Build history of the part. All positions in model axes, mm. Give positions to 0.01 mm unless a question says otherwise; leave off trailing zeros. Write each loop counter-clockwise with the first axis right and the second up, starting at its lowest first coordinate (ties: lowest second). Pieces come first, ordered by that corner, then holes. Notation, with made-up numbers: M 39,-17 L 98,-17 A16 ccw 98,-13 Z; hole C 33.5,-5 d1. An arc over 180 degrees is marked long. Return JSON: item names as keys, results as strings. Group by question number.
Q1. Flat gauge pin, fed straight in: pin 1 Ø7 at (x, z) = (0, -36.591) entering from +Y. Where does the tip first touch, or does it go through?
Q2. Band-saw the part on B-B, the plane y = 6. Give the cut face in (x, z), then the cut area to 3 significant figures.
Q3. Band-saw the part on C-C, the plane z = 32. Give the cut face in (x, y).
Q4. Band-saw the part on A-A, the plane x = 0. Give the cut face in (y, z), then the cut area to 3 significant figures.
Q5. Wall check: probe 1 along Z at (x, y) = (0, 5.75); probe 2 along X at (y, z) = (3.5, -32); probe 3 along Z at (x, y) = (4.75, 0.75). Give the ranges that are in metal, low to high.
Q6. Pull direction X, two halves, no side cores. Call faces 1 (the flat face through (-9, 4, -1)), 2 (the cylindrical face through (-3.226, 4.437, -41.65)), 3 (the flat face through (0, 0, 1)): +X half, -X half, draft (parallel to the pull), parting line (faces both ways), or undercut.
Autodesk Inventor part; units mm, degrees
ref_plane "YZ Plane" through (0, 0, 0) normal (1, 0, 0) x (0, 1, 0)
ref_plane "XZ Plane" through (0, 0, 0) normal (0, 1, 0) x (-1, 0, 0)
ref_plane "XY Plane" through (0, 0, 0) normal (0, 0, 1) x (1, 0, 0)
sketch "Sketch1" plane through (0, 0, 0) normal (0, 1, 0) x (-1, 0, 0)
  line L0 (3.6, 44.409) -> (-3.6, 44.409)
  line L1 (-9, 39.009) -> (-9, -39.009)
  line L2 (-3.6, -44.409) -> (3.6, -44.409)
  line L3 (9, -39.009) -> (9, 39.009)
  line L4 (9, 44.409) -> (-9, -44.409) construction
  line L5 (-9, 44.409) -> (9, -44.409) construction
  arc A0 (3.6, -44.409) -> (9, -39.009) centre (3.6, -39.009) ccw
  arc A1 (-9, -39.009) -> (-3.6, -44.409) centre (-3.6, -39.009) ccw
  arc A2 (9, 39.009) -> (3.6, 44.409) centre (3.6, 39.009) ccw
  arc A3 (-3.6, 44.409) -> (-9, 39.009) centre (-3.6, 39.009) ccw
  line L6 (0, -44.409) -> (0, -36.591)
  circle A4 centre (0, -36.591) radius 6
  line L7 (0, 0) -> (1.5436, 0)
  circle A5 centre (0, 36.591) radius 6
  dimension "d0" = 18
  dimension "d1" = 88.818
  dimension "d2" = 5.4
  dimension "d3" = 7.818
  dimension "d4" = 12
extrude "Extrusion1" add sketch "Sketch1" along normal blind 9
properties part number "LegLverr"
From the geometry:
{
 "1": {"pin 1": "passes through"},
 "2": {"outline": "M -9,-39.01 A5.4 ccw -3.6,-44.41 L 3.6,-44.41 A5.4 ccw 9,-39.01 L 9,39.01 A5.4 ccw 3.6,44.41 L -3.6,44.41 A5.4 ccw -9,39.01 Z; hole C 0,-36.59 d12; hole C 0,36.59 d12", "area": "1,350 mm^2"},
 "3": {"outline": "M -9,0 L -3.86,0 L -3.86,9 L -9,9 Z; M 3.86,0 L 9,0 L 9,9 L 3.86,9 Z"},
 "4": {"outline": "M 0,-44.41 L 9,-44.41 L 9,-42.59 L 0,-42.59 Z; M 0,-30.59 L 9,-30.59 L 9,30.59 L 0,30.59 Z; M 0,42.59 L 9,42.59 L 9,44.41 L 0,44.41 Z", "area": "583 mm^2"},
 "5": {"probe 1": "z = -44.41 to -42.59, -30.59 to 30.59, 42.59 to 44.41", "probe 2": "x = -9 to -3.86, 3.86 to 9", "probe 3": "z = -44.29 to -40.26, -32.93 to 32.93, 40.26 to 44.29"},
 "6": {"face 1": "-X half", "face 2": "undercut", "face 3": "draft"}
}
